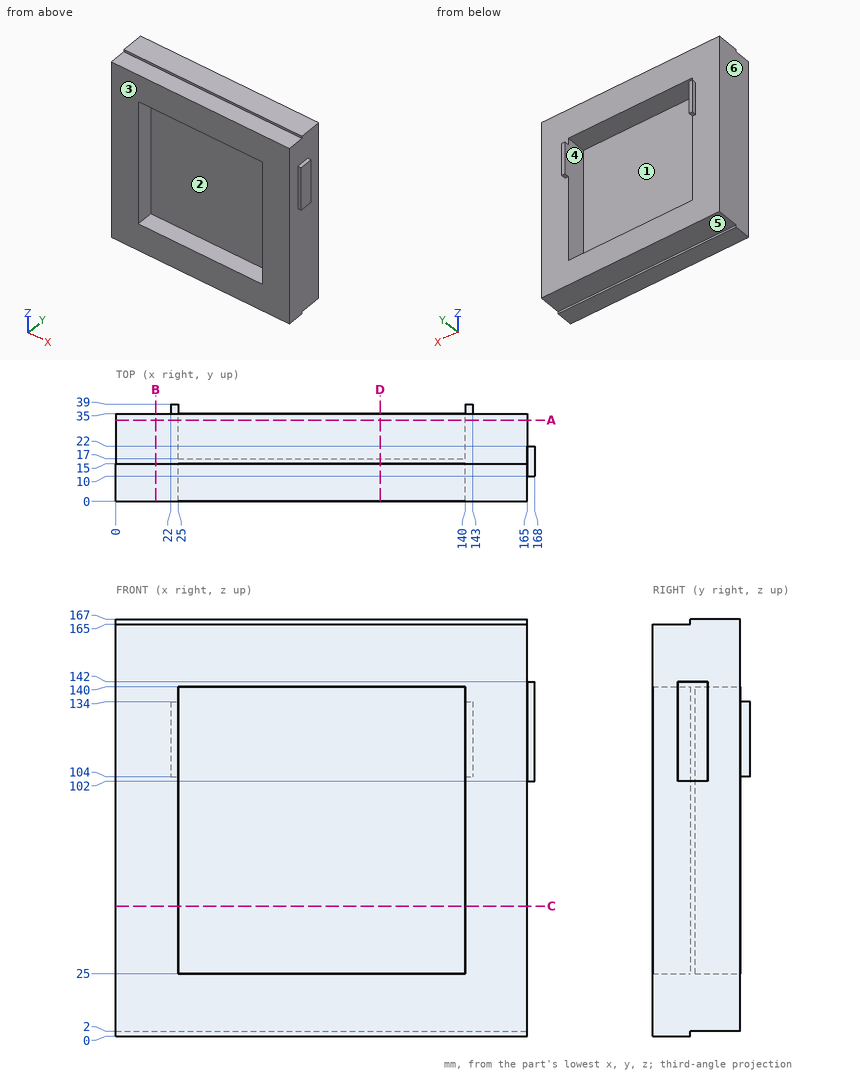
Geometry: see drawing. Coordinates: mm, zero at the bounding-box minimum. A direction names the side the tool comes from. Give positions to 0.01 mm unless a question says otherwise; leave off trailing zeros. Write each loop counter-clockwise with the first axis right and the second up, starting at its lowest first coordinate (ties: lowest second). Pieces come first, ordered by that corner, then holes. Notation, with made-up numbers: M 42,28 L 72,28 A13 cw 72,38 Z; hole C 52,21 d1. An arc over 180 degrees is marked long. Return JSON: item names as keys, results as strings. Group by question number.
1) First-contact query: pin 1 Ø8 at (x, z) = (25, 141.5) entering from -Y; pin 2 Ø6 at (x, y) = (62.5, 30) entering from -Z; pin 3 Ø0.9 at (x, y) = (142, 36.5) entering from +Z; pin 4 Ø1.5 at (x, z) = (118, 139) entering from -Y. Flat tips, straight axial feed; report the tip coordinate or a pass-through.
2) Cut plane A-A, the plane y = 32.5. Output: boundary loops of the cut face in (x, z), then the cut area to 3 significant figures.
3) Cut plane C-C, the plane z = 52. Output: boundary loops of the cut face in (x, y).
4) Cut plane D-D, the plane x = 106. Output: boundary loops of the cut face in (y, z).
5) Draft query along X for the marked faces 4, 5 and 6. Return one class per face: released by +X, released by -X, zero draft, split by the parting line, or undercut.
6) Cut plane B-B, the plane x = 16. Output: boundary loops of the cut face in (y, z), then the cut area to 4 significant figures.
7) Set-up query: the marked faces 1, 2 and 3. Return all of +Z, -Z, +X, -X, +Y, -Y with unobstructed straight access to the full face (end or side cutting, diameter ignored); none if empty.
8) Ray query, L1, parallel to X at y = 22.5, z = 81; L2, parallel to Z at x = 52.5, y = 23.5; L3, parallel to X at y = 11, z = 110. Return the intervals inside material, ascending.
Data:
{
 "1": {"pin 1": "stops at y = 0", "pin 2": "stops at z = 2", "pin 3": "stops at z = 134", "pin 4": "stops at y = 15"},
 "2": {"outline": "M 0,2 L 165,2 L 165,167 L 0,167 Z; hole M 25,25 L 140,25 L 140,140 L 25,140 Z", "area": "14,000 mm²"},
 "3": {"outline": "M 0,0 L 25,0 L 25,15 L 140,15 L 140,0 L 165,0 L 165,35 L 140,35 L 140,17 L 25,17 L 25,35 L 0,35 Z"},
 "4": {"outline": "M 0,0 L 15,0 L 15,2 L 35,2 L 35,25 L 17,25 L 17,140 L 35,140 L 35,167 L 15,167 L 15,165 L 0,165 L 0,140 L 15,140 L 15,25 L 0,25 Z"},
 "5": {"face 4": "undercut", "face 5": "zero draft", "face 6": "released by -X"},
 "6": {"outline": "M 0,0 L 15,0 L 15,2 L 35,2 L 35,167 L 15,167 L 15,165 L 0,165 Z", "area": "5,775 mm²"},
 "7": {"face 1": "+Y", "face 2": "-Y", "face 3": "+Z, -Z, +X, -X, -Y"},
 "8": {"L1": "x = 0 to 25, 140 to 165", "L2": "z = 2 to 25, 140 to 167", "L3": "x = 0 to 25, 140 to 168"}
}
